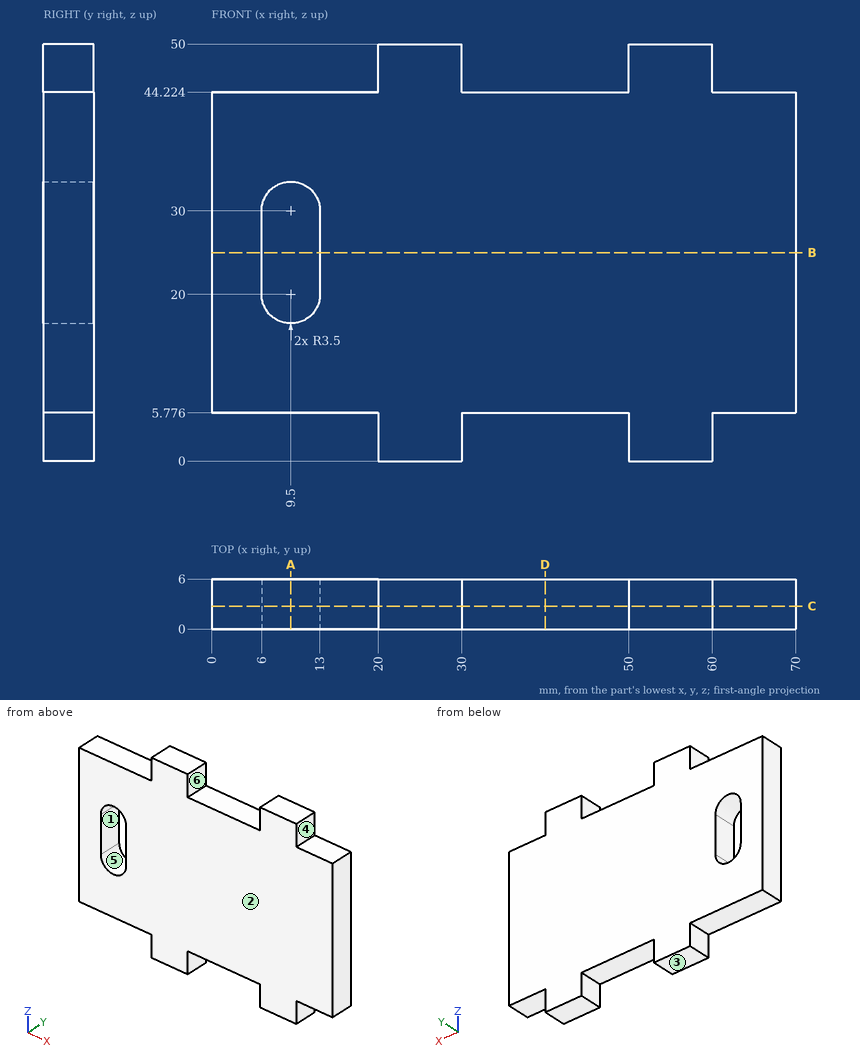
The drawing under review shows one solid part. Ordinate dimensions are in mm from its lowest x, y, z. A direction names the side the tool comes from. Give positions to 0.01 mm unless a question says otherwise; leave off trailing zeros. Loops run counter-clockwise (first coordinate to the right, second up) from the corner with the lowest first, then second, coordinate; pieces in that order, holes last. Notation, with made-up numbers: M 9,8.25 L 46,8.25 A23 ccw 46,23.25 Z; hole C 55,39 d2. An arc over 180 degrees is marked long. Return JSON: item names as keys, results as strings. Group by question number.
Item 1: We need section D-D (x = 40). Give the boundary of the cut face in (y, z) (1 decimal), and give its area (3 significant figures).
Item 2: For probe 1 along X at (y, z) = (2.1, 45); probe 2 along X at (y, z) = (5.25, 25); probe 3 along Z at (x, y) = (35.5, 4.35) (1 decimal), list the stretches that pass through material, from the lowest coordinate up.
Item 3: We need section C-C (y = 2.75). Give the boundary of the cut face in (x, z) (1 decimal).
Item 4: We need section A-A (x = 9.5). Give the boundary of the cut face in (y, z) (1 decimal).
Item 5: Mouldability with a two-part tool opening along Z and no side actions: class the marked faces 1, 2 and 3 as released by +Z, released by -Z, zero draft, split by the parting line, or undercut.
Item 6: We need section B-B (z = 25). Give the boundary of the cut face in (x, y), and give its area (3 significant figures).
Item 7: Insertion check: pin 1 Ø1.7 at (y, z) = (3.5, 48.5) entering from -X; pin 2 Ø1.7 at (y, z) = (4, 4) entering from +X; pin 3 Ø1.8 at (x, y) = (64, 3.5) entering from -Z. Each pin has a flat end and moves straight along its axis. Give the tip position at first contact, or say it passes through.
Item 8: Tool access review of the marked faces 4, 5 and 6: name each direction out of +Z, -Z, +X, -X, +Y, -Y from which nothing blocks a thin tool from reaching the whole face with its end or side.
Output:
{
 "1": {"outline": "M 0,5.8 L 6,5.8 L 6,44.2 L 0,44.2 Z", "area": "231 mm^2"},
 "2": {"probe 1": "x = 20 to 30, 50 to 60", "probe 2": "x = 0 to 6, 13 to 70", "probe 3": "z = 5.8 to 44.2"},
 "3": {"outline": "M 0,5.8 L 20,5.8 L 20,0 L 30,0 L 30,5.8 L 50,5.8 L 50,0 L 60,0 L 60,5.8 L 70,5.8 L 70,44.2 L 60,44.2 L 60,50 L 50,50 L 50,44.2 L 30,44.2 L 30,50 L 20,50 L 20,44.2 L 0,44.2 Z; hole M 6,20 A3.5 ccw 13,20 L 13,30 A3.5 ccw 6,30 Z"},
 "4": {"outline": "M 0,5.8 L 6,5.8 L 6,16.5 L 0,16.5 Z; M 0,33.5 L 6,33.5 L 6,44.2 L 0,44.2 Z"},
 "5": {"face 1": "undercut", "face 2": "zero draft", "face 3": "released by -Z"},
 "6": {"outline": "M 0,0 L 6,0 L 6,6 L 0,6 Z; M 13,0 L 70,0 L 70,6 L 13,6 Z", "area": "378 mm^2"},
 "7": {"pin 1": "stops at x = 20", "pin 2": "stops at x = 60", "pin 3": "stops at z = 5.78"},
 "8": {"face 4": "+Z, +X, +Y, -Y", "face 5": "+Y, -Y", "face 6": "+Z, +Y, -Y"}
}
